from build123d import *

# Parameters (mm, degrees)
SKETCH1_W           = 40
SKETCH1_H           = 20
BOSS_EXTRUDE1_DEPTH = 35
SKETCH2_W           = 50
SKETCH2_H           = 30
SKETCH2_W_2         = 44
SKETCH2_H_2         = 24
BOSS_EXTRUDE2_DEPTH = 35
SKETCH3_W           = 70
SKETCH3_H           = 60
BOSS_EXTRUDE4_DEPTH = 3
SKETCH6_W           = 40
SKETCH6_H           = 20
CUT_EXTRUDE1_DEPTH  = 35


with BuildPart() as part:
    # Sketch1 → Boss-Extrude1 (new body)
    with BuildSketch(Plane(origin=(0, 0, 0), x_dir=(1, 0, 0), z_dir=(0, 1, 0))):
        Rectangle(SKETCH1_W, SKETCH1_H)
    extrude(amount=BOSS_EXTRUDE1_DEPTH)



with BuildPart() as body_2:
    # Sketch2 → Boss-Extrude2 (new body)
    with BuildSketch(Plane(origin=(0, 0, 0), x_dir=(1, 0, 0), z_dir=(0, 1, 0))):
        Rectangle(SKETCH2_W, SKETCH2_H)
        Rectangle(SKETCH2_W_2, SKETCH2_H_2, mode=Mode.SUBTRACT)
    extrude(amount=BOSS_EXTRUDE2_DEPTH)


with BuildPart() as part_1:
    add(part.part)

    add(body_2.part)  # Boss-Extrude4 merges body 2
    # Sketch3 → Boss-Extrude4 (add)
    with BuildSketch(Plane.XZ):
        with Locations((10, 0)):
            Rectangle(SKETCH3_W, SKETCH3_H)
    extrude(amount=BOSS_EXTRUDE4_DEPTH)

    # Sketch6 → Cut-Extrude1 (cut)
    with BuildSketch(Plane(origin=(0, 35, 0), x_dir=(1, 0, 0), z_dir=(0, 1, 0))):
        Rectangle(SKETCH6_W, SKETCH6_H)
    extrude(amount=-CUT_EXTRUDE1_DEPTH, mode=Mode.SUBTRACT)


solid = part_1.part
Could you check a few things on this model? Use its own coordinates, in mm. A direction names the side the tool comes from. Round coordinates to 2 decimals unless told otherwise and drop trailing zeros. Loops run counter-clockwise (first coordinate to the right, second up) from the corner with the lowest first, then second, coordinate; pieces in that order, holes last. Notation, with made-up numbers: (-16.75, 66.5) - (-11.75, 66.5) arc R20 cw to (-11.75, 89.5) - close; hole circle Ø1 at (20, 5.5). An arc over 180 degrees is marked (long way). Write item = value, one per line.
1) Imagine slicing it at C-C (z = -8). Please give me the cut outline in (x, y).
Computed:
outline = (-25, -3) - (45, -3) - (45, 0) - (25, 0) - (25, 35) - (22, 35) - (22, 0) - (-22, 0) - (-22, 35) - (-25, 35) - close
2) I'm going to push flat-ended pins straight in: P1, Ø2, axis at y = 28, z = 9.5, coming from the +X side; P2, Ø17.5, axis at x = -9.5, y = 19, coming from the -Z side; P3, Ø12, axis at x = 37.5, z = -2, coming from the +Y side. Where does each tip first touch, or does it pass through?
Computed:
P1 = 25
P2 = -15
P3 = 0
3) Imagine slicing it at B-B (x = 1). Please give me the cut outline in (y, z), and give its area (3 significant figures).
Computed:
outline = (-3, -30) - (0, -30) - (0, -15) - (35, -15) - (35, -12) - (0, -12) - (0, 12) - (35, 12) - (35, 15) - (0, 15) - (0, 30) - (-3, 30) - close
area = 390 mm2
4) Imagine slicing it at D-D (z = -16). Please give me the cut outline in (x, y), and give its area (3 significant figures).
Computed:
outline = (-25, -3) - (45, -3) - (45, 0) - (-25, 0) - close
area = 210 mm2
5) On a 3-axis mill with a long thin cutter (end or side, diameter ignored), from which of +Z, -Z, +X, -X, +Y, -Y can I reach the whole of each face in a straight line? I mean faces 4 (the flat face through (0, 17, -12)), 5 (the flat face through (0, 17, 15)), 6 (the flat face through (10, -3, 0)), 7 (the flat face through (0, 17, -15)), 8 (the flat face through (25, 17, 0)). Say none if no direction works.
Computed:
face_4 = +Y
face_5 = +Z, +X, -X, +Y
face_6 = +Z, -Z, +X, -X, -Y
face_7 = -Z, +X, -X, +Y
face_8 = +Z, -Z, +X, +Y
6) I need wall thicknesses on line 1 along X through (y, z) = (15.5, -11.5); line 2 along Z through (x, y) = (2.5, 16); line 3 along Y through (x, z) = (15, 8.5). Which ranges of each line are inside material? Lowest first, please. Write a range as from..to.
Computed:
line_1 = -25..-22, 22..25
line_2 = -15..-12, 12..15
line_3 = -3..0
7) Imagine slicing it at A-A (y = 18.5). Please give me the cut outline in (x, z).
Computed:
outline = (-25, -15) - (25, -15) - (25, 15) - (-25, 15) - close; hole (-22, -12) - (22, -12) - (22, 12) - (-22, 12) - close
8) If we mould it in two halves opening along X, with no side actions, what happens to faces 1 (the flat face through (-25, 16, 0)), 2 (the flat face through (10, -1, -30)), 3 (the flat face through (0, 17, 12))? For each: pulls with the +X half, pulls with the -X half, needs draft (parallel to the pull), parting line crosses it, or undercut.
Computed:
face_1 = pulls with the -X half
face_2 = needs draft
face_3 = undercut
